CAD build for the part. Positions are in the model's coordinates, mm. A direction names the side the tool comes from. Give positions to 0.01 mm unless a question says otherwise; leave off trailing zeros. Write each loop counter-clockwise with the first axis right and the second up, starting at its lowest first coordinate (ties: lowest second). Pieces come first, ordered by that corner, then holes. Notation, with made-up numbers: (18, 3) - (46, 3) arc R16 cw to (46, 26) - close; hole circle Ø7 at (68, 32.5). An arc over 180 degrees is marked (long way). Answer as a JSON object with one key per item and string values.
from build123d import *

# Parameters (mm, degrees)
F0_W      = 50
F0_H      = 12.5
F1_DEPTH  = 8
F2_DEPTH  = 75
F4_DEPTH  = 8
F7_DEPTH  = 3
F8_DEPTH  = 1
F11_DEPTH = 3
F14_DEPTH = 3
F15_DEPTH = 8
F16_DEPTH = 8
F17_DEPTH = 12.5


with BuildPart() as f1:
    # F0 (on Top) → F1 (new body)
    with BuildSketch(Plane.XY):
        Polygon((42.017949, -72.777223), (84.035898, 0), (42.017949, 72.777223), (-42.017949, 72.777223), (-84.035898, 0), (-42.017949, -72.777223), align=None)
        with Locations((0, 54.582917)):
            Rectangle(F0_W, F0_H, mode=Mode.SUBTRACT)
    extrude(amount=F1_DEPTH)

    # F0 (on Top) → F2 (join)
    with BuildSketch(Plane.XY):
        Polygon((68.124673, -33.55905), (87.5, 0), (84.035898, 0), (42.017949, -72.777223), (-42.017949, -72.777223), (-84.035898, 0), (-87.5, 0), (-68.124673, -33.55905), (-63.174512, -42.132981), (-43.75, -75.777223), (43.75, -75.777223), (63.174512, -42.132981), align=None)
    extrude(amount=F2_DEPTH)

    # F0 (on Top) → F4 (join)
    with BuildSketch(Plane.XY):
        Polygon((43.75, 75.777223), (-43.75, 75.777223), (-65.625, 37.888611), (-68.125, 33.558484), (-87.5, 0), (-84.035898, 0), (-42.017949, 72.777223), (42.017949, 72.777223), (84.035898, 0), (87.5, 0), align=None)
    extrude(amount=F4_DEPTH)

    # F6 (on face) → F7 (join)
    with BuildSketch(Plane(origin=(0, -50.131237, 89.383668), x_dir=(1, 0, 0), z_dir=(0, 0.489171, -0.872188))):
        Polygon((43.75, 29.404192), (0, 29.404192), (-43.75, 29.404192), (-42.01795, -57.477552), (42.01795, -57.477552), align=None)
    extrude(amount=F7_DEPTH)

    # F3 (on Front) → F8 (join)
    with BuildSketch(Plane.XZ):
        Polygon((-42.01795, 114.5), (0, 114.5), (42.01795, 114.5), (84.0359, 75), (87.5, 75), (42.01795, 117.5), (0, 117.5), (-42.01795, 117.5), (-87.5, 75), (-84.0359, 75), align=None)
    extrude(amount=F8_DEPTH)

    # F10 (on face) → F11 (join)
    with BuildSketch(Plane(origin=(-67.684673, -39.077764, 72.433827), x_dir=(0.772363, -0.301588, 0.559017), z_dir=(-0.635181, -0.366722, 0.67975))):
        Polygon((33.231426, 55.789645), (-25.65546, 35.610412), (30.988892, -31.080422), align=None)
    extrude(amount=-F11_DEPTH)

    # F13 (on face) → F14 (join)
    with BuildSketch(Plane(origin=(67.675669, -39.595085, 72.424192), x_dir=(0.773305, 0.304147, -0.556322), z_dir=(-0.634035, 0.370955, -0.678522))):
        Polygon((-30.93951, 30.511739), (-32.875165, -56.364915), (25.940007, -35.977606), align=None)
    extrude(amount=F14_DEPTH)

    # F0 (on Top) → F15 (join)
    with BuildSketch(Plane.XY):
        with Locations((0, 54.582917)):
            Rectangle(F0_W, F0_H)
    extrude(amount=F15_DEPTH)

    # F0 (on Top) → F16 (join)
    with BuildSketch(Plane.XY):
        Polygon((-78.447809, -39.67729), (-73.329958, -36.64408), (-75.878554, -32.343907), (-80.946091, -35.46201), align=None)
        Polygon((-63.174512, -42.132981), (-68.124673, -33.55905), (-73.329958, -36.64408), (-78.447809, -39.67729), (-73.398516, -48.192843), (-68.261641, -45.14817), align=None)
        Polygon((-65.73638, -49.405581), (-68.261641, -45.14817), (-73.398516, -48.192843), (-70.880193, -52.396181), align=None)
        Polygon((75.878554, -32.343907), (73.329958, -36.64408), (78.447809, -39.67729), (80.946091, -35.46201), align=None)
        Polygon((73.329958, -36.64408), (68.124673, -33.55905), (63.174512, -42.132981), (68.261641, -45.14817), (73.398516, -48.192843), (78.447809, -39.67729), align=None)
        Polygon((73.398516, -48.192843), (68.261641, -45.14817), (65.73638, -49.405581), (70.880193, -52.396181), align=None)
    extrude(amount=F16_DEPTH)

    # F0 (on Top) → F17 (cut, symmetric)
    with BuildSketch(Plane.XY):
        with Locations((0, 54.582917)):
            Rectangle(F0_W, F0_H)
    extrude(amount=F17_DEPTH, both=True, mode=Mode.SUBTRACT)


solid = f1.part
(1) Probe L1, parallel to Y at x = 41, z = 39; L2, parallel to Z at x = -43.5, y = 14; L3, parallel to X at y = -13, z = 10. List the from-to ranges inside material, lowest first. Write a range as [from, to].
Answer key:
{"L1": "y = [-75.78, -72.78]", "L2": "z = [0, 8]", "L3": "x = [-79.99, -76.53], [76.53, 79.99]"}
(2) Flat gauge pins, fed straight in: P1, Ø2, axis at x = 26.5, z = 91.5, coming from the +Y side; P2, Ø3.5, axis at x = 84, z = 78.5, coming from the +Y side; P3, Ø5.5, axis at x = -70.5, y = -45, coming from the +Z side. Where does each tip first touch, or does it go through?
Answer key:
{"P1": "stops at y = -38.44", "P2": "stops at y = 0.63", "P3": "stops at z = 8"}
(3) Saw through at D-D, the plane y = 54. Give the cut face in (x, z).
Answer key:
{"outline": "(-56.32, 0) - (-25, 0) - (-25, 8) - (-56.32, 8) - close; (25, 0) - (56.32, 0) - (56.32, 8) - (25, 8) - close"}
(4) Pull direction X, two halves, no side cores. Call faces 6 (the face through (-68.34, -50.92, 3.94)), 7 (the face through (-0.613, -38.912, 95.676)), 8 (the face through (65.93, 37.36, 3.94)): pulls with the +X half, pulls with the -X half, needs draft (parallel to the pull), parting line crosses it, or undercut.
Answer key:
{"face 6": "undercut", "face 7": "needs draft", "face 8": "pulls with the +X half"}
(5) Saw through at B-B, the plane z = 31.5. Give the cut face in (x, y).
Answer key:
{"outline": "(-87.5, 0) - (-43.75, -75.78) - (43.75, -75.78) - (87.5, 0) - (84.04, 0) - (42.02, -72.78) - (-42.02, -72.78) - (-84.04, 0) - close"}
(6) 3-axis set-ups, long thin cutter, end or side, ignore diameter. For faces 1 (the face through (-1, -75.777, 37)), 2 (the face through (78.448, -33.925, 3.944)), 3 (the face through (0, 60.833, 4)), 4 (the face through (54.57, -25.47, 92.39)), 5 (the face through (-53.7, -22, 90.3)): which of +Z, -Z, +X, -X, +Y, -Y reach the whole face in a straight line?
Answer key:
{"face 1": "+Z, -Z, +X, -X, -Y", "face 2": "+Z, -Z, +X", "face 3": "+Z, -Z", "face 4": "+Z, +X, -Y", "face 5": "+Y"}
